from build123d import *

# Parameters (mm, degrees)
SKETCH122_R           = 1.7
PAD049_DEPTH          = 6
SKETCH123_R           = 19
SKETCH123_R_2         = 14.5
PAD050_DEPTH          = 27
POCKET086_DEPTH       = 14
SKETCH125_R           = 0.886763
POCKET087_DEPTH       = 10
POLARPATTERN004_COUNT = 4
SKETCH150_R           = 19
PAD063_DEPTH          = 2


with BuildPart() as part:
    # Sketch122 → Pad049 (new body)
    with BuildSketch(Plane.XY):
        Polygon((8.427001, 21.382204), (-8.425608, 21.382204), (-19.924648, 11.454167), (-19.507777, -12.150562), (-8.24189, -21.453689), (8.242053, -21.453689), (44.039975, -7.608119), (48.125982, -2.870427), (48.125982, 2.870427), (43.951076, 7.65457), align=None)
        with Locations((40.008084, 0)):
            Circle(SKETCH122_R, mode=Mode.SUBTRACT)
        with BuildLine():
            ThreePointArc((14.231577, 2.509486), (10.260151, 10.176669), (2.625669, 14.210601))
            Line((2.625669, 17.896729), (2.625669, 14.210601))
            Line((-2.582623, 17.896729), (2.625669, 17.896729))
            Line((-2.582682, 14.218476), (-2.582623, 17.896729))
            ThreePointArc((-2.582682, 14.218476), (-10.244752, 10.192172), (-14.231577, 2.509486))
            Line((-17.812584, 2.509486), (-14.231577, 2.509486))
            Line((-17.812584, -2.46093), (-17.812584, 2.509486))
            Line((-14.240297, -2.459525), (-17.812584, -2.46093))
            ThreePointArc((-14.240297, -2.459525), (-10.262224, -10.174579), (-2.581573, -14.218677))
            Line((-2.581573, -17.991852), (-2.581573, -14.218677))
            Line((2.625669, -17.991852), (-2.581573, -17.991852))
            Line((2.625669, -14.210601), (2.625669, -17.991852))
            ThreePointArc((2.625669, -14.210601), (10.277853, -10.158791), (14.240229, -2.459917))
            Line((17.937973, -2.459917), (14.240229, -2.459917))
            Line((17.937973, 2.509486), (17.937973, -2.459917))
            Line((14.231577, 2.509486), (17.937973, 2.509486))
        make_face(mode=Mode.SUBTRACT)
        with BuildLine():
            ThreePointArc((24.762929, 9.570019), (22.008084, 0), (24.762929, -9.570019))
            ThreePointArc((24.762929, -9.570019), (26.937298, -9.618098), (26.985377, -7.443729))
            ThreePointArc((26.985377, 7.443729), (25.008084, 0), (26.985377, -7.443729))
            ThreePointArc((26.985377, 7.443729), (26.937298, 9.618098), (24.762929, 9.570019))
        make_face(mode=Mode.SUBTRACT)
    extrude(amount=PAD049_DEPTH)

    # Sketch123 (on Face32 of Pad049) → Pad050 (join)
    with BuildSketch(Plane(origin=(0, 0, 0), x_dir=(1, 0, 0), z_dir=(0, 0, -1))):
        Circle(SKETCH123_R)
        Circle(SKETCH123_R_2, mode=Mode.SUBTRACT)
    extrude(amount=PAD050_DEPTH)

    # Sketch124 (on Face35 of Pad050) → Pocket086 (cut)
    with BuildSketch(Plane(origin=(0, 0, -27), x_dir=(1, 0, 0), z_dir=(0, 0, -1))):
        Polygon((0, 0), (-42.583396, 24.585535), (42.583396, 24.585535), align=None)
    extrude(amount=-POCKET086_DEPTH, mode=Mode.SUBTRACT)

    # Sketch125 (on Face44 of Pocket086) → Pocket087 (cut)
    with BuildSketch(Plane.XY):
        with Locations((0, 15.490395)):
            Circle(SKETCH125_R)
    pocket087 = extrude(amount=-POCKET087_DEPTH, mode=Mode.SUBTRACT)

    # PolarPattern004: Pocket087 ×4 about axis
    polarpattern004_axis = Axis((0, 0, 0), (0, 0, 1))
    for i in range(1, POLARPATTERN004_COUNT):
        add(pocket087.rotate(polarpattern004_axis, i * 360 / POLARPATTERN004_COUNT), mode=Mode.SUBTRACT)

    # Sketch150 (on Face35 of PolarPattern004) → Pad063 (join)
    with BuildSketch(Plane(origin=(0, 0, -27), x_dir=(1, 0, 0), z_dir=(0, 0, -1))):
        Circle(SKETCH150_R)
    extrude(amount=PAD063_DEPTH)


with BuildPart() as part_1:
    # Body023 placement: moved
    add(part.part.moved(Location((0, 66, 21))))


solid = part_1.part
Could you check a few things on this model? Use its own coordinates, in mm. A direction names the side the tool comes from. Give positions to 0.01 mm unless a question says otherwise; leave off trailing zeros. Order: outer loops, then holes, each group sorted by start corner. A loop starts at its lowest first (then second) coordinate and runs counter-clockwise, first axis right, second up. Notation, with made-up numbers: (-23, 38.25) - (24, 38.25) arc R18 cw to (24, 58.25) - close; hole circle Ø6 at (78.5, -39.75). An arc over 180 degrees is marked (long way). Return JSON: item names as keys, results as strings. Group by question number.
Q1. Thinking about a two-plate mould opening in X: for faces 1 (the face through (21, 66, 21)), 2 (the face through (14.951, 66.704, 16.07)), which applies, pulls with the +X half, pulls with the -X half, needs draft (parallel to the pull), parting line crosses it, or undercut?
Q2. Please list where these lines run through material, in increasing order: line 1 along Y through (x, z) = (0, 10.5); line 2 along Z through (x, y) = (-1, 50); line 3 along Z through (x, y) = (27, 66.5). Write a range as [from, to].
Q3. Suppose I cut it at C-C, the plane y = 60.5. Please give me the cut outline in (x, z), and give its area (3 significant figures).
Q4. Suppose I cut it at A-A, the plane x = 0. Please give me the cut outline in (y, z).
Q5. Which directions (+Z, -Z, +X, -X, +Y, -Y) give clear straight access to the entire face, cutting with the end or side of a thin tool? Please do faces 3 (the face through (22.01, 66.14, 23.96)), 4 (the face through (14, 71, 27)), 5 (the face through (-17.813, 66, 24)).
Q6. Suppose I cut it at B-B, the plane z = 23.5. State how many separate pieces and enclosed holes the cut face has, and give its area (3 significant figures).
Q7. Will these pins go through, and if not, where does the flat tip stop? pin 1 Ø1.6 at (x, y) = (15.49, 66) entering from +Z; pin 2 Ø10 at (x, z) = (18.5, 15) entering from -Y; pin 3 Ø3 at (x, z) = (28, 20.5) entering from +Y.
Resolved:
{
 "1": {"face 1": "needs draft", "face 2": "undercut"},
 "2": {"line 1": "y = [47, 51.5], [80.5, 85]", "line 2": "z = [-8, -6], [8, 21]", "line 3": "z = [21, 27]"},
 "3": {"outline": "(-19.63, 21) - (-18.19, 21) - (-18.19, -8) - (18.19, -8) - (18.19, 21) - (22.87, 21) - (22.87, 27) - (13.36, 27) - (13.36, 21) - (13.42, 21) - (13.42, -6) - (-13.42, -6) - (-13.42, 21) - (-13.36, 21) - (-13.36, 27) - (-19.63, 27) - close; (26.05, 21) - (45.86, 21) - (45.86, 27) - (26.05, 27) - close", "area": "544 mm2"},
 "4": {"outline": "(44.55, 21) - (47, 21) - (47, 8) - (51.5, 8) - (51.5, 21) - (51.4, 21) - (51.4, 11) - (49.62, 11) - (49.62, 21) - (48.01, 21) - (48.01, 27) - (44.55, 27) - close; (47, -8) - (85, -8) - (85, 21) - (87.38, 21) - (87.38, 27) - (83.9, 27) - (83.9, 21) - (82.38, 21) - (82.38, 11) - (80.6, 11) - (80.6, 21) - (80.5, 21) - (80.5, -6) - (47, -6) - close"},
 "5": {"face 3": "+Z, -Z", "face 4": "+Z, +X, -X, +Y, -Y", "face 5": "+Z"},
 "6": {"separate pieces": "1", "enclosed holes": "3", "area": "1,370 mm2"},
 "7": {"pin 1": "stops at z = 11", "pin 2": "stops at y = 52.63", "pin 3": "stops at y = 80.37"}
}
